from build123d import *

# Parameters (mm, degrees)
SKETCH_W        = 19.05
SKETCH_H        = 9.525
PAD_DEPTH       = 469.9
SKETCH001_W     = 9.525
SKETCH001_H     = 2.38125
POCKET_DEPTH    = 469.901
SKETCH002_W     = 14.2875
SKETCH002_H     = 3.175
POCKET001_DEPTH = 469.901
SKETCH003_W     = 11.1125
SKETCH003_H     = 1.5875
POCKET002_DEPTH = 469.901


with BuildPart() as part:
    # Sketch → Pad (new body)
    with BuildSketch(Plane.XZ):
        Rectangle(SKETCH_W, SKETCH_H)
    extrude(amount=PAD_DEPTH)

    # Sketch001 (on Face6 of Pad) → Pocket (cut, through all)
    with BuildSketch(Plane.XZ.offset(469.9)):
        with Locations((0, 3.571875)):
            Rectangle(SKETCH001_W, SKETCH001_H)
    extrude(amount=-POCKET_DEPTH, mode=Mode.SUBTRACT)

    # Sketch002 (on Face5 of Pocket) → Pocket001 (cut, through all)
    with BuildSketch(Plane.XZ.offset(469.9)):
        with Locations((0, 0.79375)):
            Rectangle(SKETCH002_W, SKETCH002_H)
    extrude(amount=-POCKET001_DEPTH, mode=Mode.SUBTRACT)

    # Sketch003 (on Face5 of Pocket001) → Pocket002 (cut, through all)
    with BuildSketch(Plane.XZ.offset(469.9)):
        with Locations((0, -1.5875)):
            Rectangle(SKETCH003_W, SKETCH003_H)
    extrude(amount=-POCKET002_DEPTH, mode=Mode.SUBTRACT)


solid = part.part
Can you work these out from the model? Positions are in its coordinate system, mm. Round coordinates to 2 decimals unless told otherwise and drop trailing zeros. Write each loop counter-clockwise with the first axis right and the second up, starting at its lowest first coordinate (ties: lowest second). Pieces come first, ordered by that corner, then holes. Notation, with made-up numbers: (72.5, 60) - (116.5, 60) arc R22 ccw to (116.5, 66) - close; hole circle Ø9 at (85, -26). An arc over 180 degrees is marked (long way). Write each question's results on one line, items separated by ' | '. Start each with the question number.
1) Suppose I cut it at A-A (y = -38.5). List the corners of the cut face in (x, z) for me (1 decimal).
2) For pin 1 Ø1 at (x, y) = (-1, -398.5) entering from +Z; pin 2 Ø2 at (x, z) = (-4.5, -1) entering from +Y, each with a flat end and sliding along its axis, tell me the tip position at first contact or that it passes through.
3) We'd pull the mould along X, two halves only. Please class faces 1 (the flat face through (9.525, -232, 0)), 2 (the flat face through (0, -238, -2.381)), 3 (the flat face through (-9.525, -232, 0)): released by +X, released by -X, zero draft, split by the parting line, or undercut.
4) Suppose I cut it at B-B (x = 1.5). List the corners of the cut face in (y, z) for me, and give its area (3 significant figures).
5) Please list where these lines run through material, in increasing order: line 1 (X direction, y = -369, z = -2) (3 decimals); line 2 (X direction, y = -150.5, z = 2) (3 decimals); line 3 (Z direction, x = 6.5, y = -340).
Here are the results:
1) outline: (-9.5, -4.8) - (9.5, -4.8) - (9.5, 4.8) - (4.8, 4.8) - (4.8, 2.4) - (7.1, 2.4) - (7.1, -0.8) - (5.6, -0.8) - (5.6, -2.4) - (-5.6, -2.4) - (-5.6, -0.8) - (-7.1, -0.8) - (-7.1, 2.4) - (-4.8, 2.4) - (-4.8, 4.8) - (-9.5, 4.8) - close
2) pin 1: stops at z = -2.38 | pin 2: passes through
3) face 1: released by +X | face 2: undercut | face 3: released by -X
4) outline: (-469.9, -4.76) - (0, -4.76) - (0, -2.38) - (-469.9, -2.38) - close | area: 1,120 mm2
5) line 1: x = -9.525 to -5.556, 5.556 to 9.525 | line 2: x = -9.525 to -7.144, 7.144 to 9.525 | line 3: z = -4.76 to -0.79, 2.38 to 4.76
